Build history of the part. All positions in model axes, mm. Coordinates: 2 decimals unless noted, no trailing zeros. Order: outer loops, then holes, each group sorted by start corner. A loop starts at its lowest first (then second) coordinate and runs counter-clockwise, first axis right, second up. Notation, with made-up numbers: M -35.75,7 L -26.75,7 A29 cw -26.75,43 Z; hole C 45,28 d9. An arc over 180 degrees is marked long. Use a Markdown table: item, result. Add a question column.
from build123d import *

# Parameters (mm, degrees)
EXTRUDE_1_DEPTH     = 2
CUT_EXTRUDE_2_REACH = 124.303
SKETCH_3_R          = 1.6
SKETCH_3_W          = 16
SKETCH_3_H          = 16
CUT_EXTRUDE_4_REACH = 124.303
SKETCH_5_R          = 1.6
FILLET_1_R          = 2
SKETCH_6_W          = 25
SKETCH_6_H          = 15
CUT_EXTRUDE_5_DEPTH = 123.302902664
CUT_EXTRUDE_6_DEPTH = 123.302902664


with BuildPart() as part:
    # 草图1 → 凸台-拉伸1 (new body)
    with BuildSketch(Plane.XY):
        Polygon((-77, 65), (77, 65), (77, -65), (77, -95), (40, -95), (40, -52), (53, -52), (53, -42), (3, -42), (3, -37), (-15, -37), (-15, -52), (-40, -52), (-40, -95), (-77, -95), (-77, -65), align=None)
    extrude(amount=EXTRUDE_1_DEPTH)

    # 草图3 → 切除-拉伸2 (cut, up to next)
    with BuildSketch(Plane.XY.offset(2), mode=Mode.PRIVATE) as cut_extrude_2_sk1:
        with Locations((-66.5, 15)):
            Circle(SKETCH_3_R)
    cut_extrude_2_tool1 = extrude(cut_extrude_2_sk1.sketch, amount=-CUT_EXTRUDE_2_REACH, mode=Mode.PRIVATE) & part.part
    # 草图3 → 切除-拉伸2 (cut, up to next)
    with BuildSketch(Plane.XY.offset(2), mode=Mode.PRIVATE) as cut_extrude_2_sk2:
        with Locations(Location((-41.5, 15, 0), (0, 0, 180))):
            Circle(SKETCH_3_R)
    cut_extrude_2_tool2 = extrude(cut_extrude_2_sk2.sketch, amount=-CUT_EXTRUDE_2_REACH, mode=Mode.PRIVATE) & part.part
    # 草图3 → 切除-拉伸2 (cut, up to next)
    with BuildSketch(Plane.XY.offset(2), mode=Mode.PRIVATE) as cut_extrude_2_sk3:
        with Locations((-54, 15)):
            Rectangle(SKETCH_3_W, SKETCH_3_H)
    cut_extrude_2_tool3 = extrude(cut_extrude_2_sk3.sketch, amount=-CUT_EXTRUDE_2_REACH, mode=Mode.PRIVATE) & part.part
    add(cut_extrude_2_tool1.solids().sort_by_distance((-66.5, 15, 2))[0], mode=Mode.SUBTRACT)
    add(cut_extrude_2_tool2.solids().sort_by_distance((-41.5, 15, 2))[0], mode=Mode.SUBTRACT)
    add(cut_extrude_2_tool3.solids().sort_by_distance((-54, 15, 2))[0], mode=Mode.SUBTRACT)

    # 草图5 → 切除-拉伸4 (cut, up to next)
    with BuildSketch(Plane.XY.offset(2), mode=Mode.PRIVATE) as cut_extrude_4_sk1:
        with Locations((72, -41.5)):
            Circle(SKETCH_5_R)
    cut_extrude_4_tool1 = extrude(cut_extrude_4_sk1.sketch, amount=-CUT_EXTRUDE_4_REACH, mode=Mode.PRIVATE) & part.part
    # 草图5 → 切除-拉伸4 (cut, up to next)
    with BuildSketch(Plane.XY.offset(2), mode=Mode.PRIVATE) as cut_extrude_4_sk2:
        with Locations((72, 51.5)):
            Circle(SKETCH_5_R)
    cut_extrude_4_tool2 = extrude(cut_extrude_4_sk2.sketch, amount=-CUT_EXTRUDE_4_REACH, mode=Mode.PRIVATE) & part.part
    # 草图5 → 切除-拉伸4 (cut, up to next)
    with BuildSketch(Plane.XY.offset(2), mode=Mode.PRIVATE) as cut_extrude_4_sk3:
        with Locations(Location((-72, 51.5, 0), (0, 0, 180))):
            Circle(SKETCH_5_R)
    cut_extrude_4_tool3 = extrude(cut_extrude_4_sk3.sketch, amount=-CUT_EXTRUDE_4_REACH, mode=Mode.PRIVATE) & part.part
    # 草图5 → 切除-拉伸4 (cut, up to next)
    with BuildSketch(Plane.XY.offset(2), mode=Mode.PRIVATE) as cut_extrude_4_sk4:
        with Locations(Location((-72, -41.5, 0), (0, 0, 180))):
            Circle(SKETCH_5_R)
    cut_extrude_4_tool4 = extrude(cut_extrude_4_sk4.sketch, amount=-CUT_EXTRUDE_4_REACH, mode=Mode.PRIVATE) & part.part
    add(cut_extrude_4_tool1.solids().sort_by_distance((72, -41.5, 2))[0], mode=Mode.SUBTRACT)
    add(cut_extrude_4_tool2.solids().sort_by_distance((72, 51.5, 2))[0], mode=Mode.SUBTRACT)
    add(cut_extrude_4_tool3.solids().sort_by_distance((-72, 51.5, 2))[0], mode=Mode.SUBTRACT)
    add(cut_extrude_4_tool4.solids().sort_by_distance((-72, -41.5, 2))[0], mode=Mode.SUBTRACT)

    # 圆角1
    fillet_1_edges = [part.edges().sort_by_distance(p)[0] for p in [
        (77, -95, 1),
        (40, -95, 1),
        (40, -52, 1),
        (53, -52, 1),
        (53, -42, 1),
        (3, -42, 1),
        (3, -37, 1),
        (-15, -37, 1),
        (-15, -52, 1),
        (-40, -52, 1),
        (-40, -95, 1),
        (-77, -95, 1),
        (-77, 65, 1),
        (77, 65, 1),
    ]]
    fillet(fillet_1_edges, radius=FILLET_1_R)

    # 草图6 → 切除-拉伸5 (cut, through all)
    with BuildSketch(Plane.XY.offset(2)):
        with Locations((47.5, 15)):
            Rectangle(SKETCH_6_W, SKETCH_6_H)
    extrude(amount=-CUT_EXTRUDE_5_DEPTH, mode=Mode.SUBTRACT)

    # 草图7 → 切除-拉伸6 (cut, through all)
    with BuildSketch(Plane.XY.offset(2)):
        with BuildLine():
            Line((-43, 53), (-20, 53))
            Line((-20, 53), (-20, 47.2))
            Line((-20, 47.2), (-15, 47.2))
            ThreePointArc((-15, 47.2), (-13.3, 45.5), (-15, 43.8))
            Line((-15, 43.8), (-20, 43.8))
            Line((-20, 43.8), (-20, 38))
            Line((-20, 38), (-43, 38))
            Line((-43, 38), (-43, 43.8))
            Line((-43, 43.8), (-48, 43.8))
            ThreePointArc((-48, 43.8), (-49.7, 45.5), (-48, 47.2))
            Line((-48, 47.2), (-43, 47.2))
            Line((-43, 47.2), (-43, 53))
        make_face()
        with BuildLine():
            Line((20, 43.8), (20, 38))
            Line((20, 38), (43, 38))
            Line((43, 38), (43, 43.8))
            Line((43, 43.8), (48, 43.8))
            ThreePointArc((48, 43.8), (49.7, 45.5), (48, 47.2))
            Line((48, 47.2), (43, 47.2))
            Line((43, 47.2), (43, 53))
            Line((43, 53), (20, 53))
            Line((20, 53), (20, 47.2))
            Line((20, 47.2), (15, 47.2))
            ThreePointArc((15, 47.2), (13.3, 45.5), (15, 43.8))
            Line((15, 43.8), (20, 43.8))
        make_face()
    extrude(amount=-CUT_EXTRUDE_6_DEPTH, mode=Mode.SUBTRACT)


solid = part.part
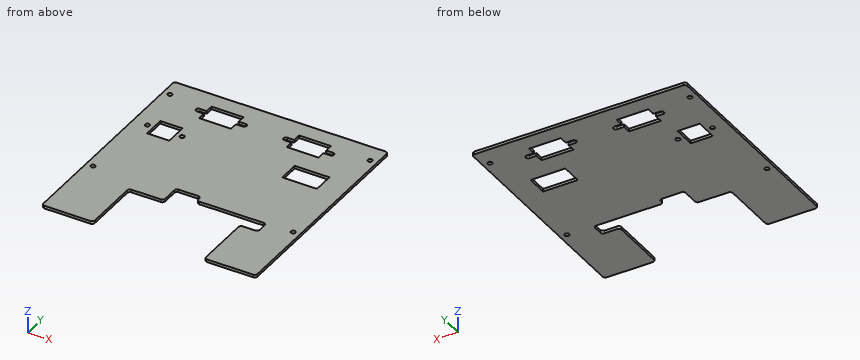
(1) Drop flat-ended pins along their axis: P1, Ø0.6, axis at x = 18, z = 1, coming from the -Y side; P2, Ø0.6, axis at x = -28.5, z = 0.5, coming from the -Y side. Give the stop position or say it passes through.
(2) Slice it at A-A on x = -25. Give the cut face in (y, z).
(3) Slice it at C-C on z = 0.35. State how many separate pieces and enclosed holes the cut face has, and give its area (3 significant figures).
(4) Slice it at B-B on y = -48. Give the cut face in (x, z).
(5) Drill centre lines: line 1 along Y through (x, z) = (-72, 1.5); line 2 along Y through (x, z) = (25, 1.5); line 3 along Y through (x, z) = (-53.5, 1.5). Where is each one in solid material? Low to high. Write a range as from..to.
Solutions:
| question | item | result |
|---|---|---|
| 1 | P1 | y = -42 |
| 1 | P2 | y = -52 |
| 2 | outline | M -52,0 L 38,0 L 38,2 L -52,2 Z; M 53,0 L 65,0 L 65,2 L 53,2 Z |
| 3 | separate pieces | 1 |
| 3 | enclosed holes | 10 |
| 3 | area | 19,000 mm² |
| 4 | outline | M -77,0 L -15,0 L -15,2 L -77,2 Z; M 53,0 L 77,0 L 77,2 L 53,2 Z |
| 5 | line 1 | -95..-43.1, -39.9..49.9, 53.1..65 |
| 5 | line 2 | -42..38, 53..65 |
| 5 | line 3 | -95..7, 23..65 |
